Autodesk Fusion 360 part; units mm, degrees
sketch "Sketch1" plane through (0, 0, 0) normal (0, 0, 1) x (1, 0, 0)
  line L0 (-21, 20) -> (67.2, 20)
  line L1 (67.2, 20) -> (67.2, -83.2)
  line L2 (67.2, -83.2) -> (-21, -83.2)
  line L3 (-21, -83.2) -> (-21, 20)
  line L4 (-24, 23) -> (70.2, 23)
  line L5 (70.2, 23) -> (70.2, -86.2)
  line L6 (70.2, -86.2) -> (-24, -86.2)
  line L7 (-24, -86.2) -> (-24, 23)
  line L8 (-21, 20) -> (-24, 20)
  line L9 (-24, 20) -> (-24, -6.1)
  line L10 (-24, -6.1) -> (-21, -6.1)
  line L11 (-21, -6.1) -> (-21, 20)
  line L12 (-21, 20) -> (-18, 20)
  line L13 (-18, 20) -> (-18, 17)
  line L14 (-18, 17) -> (-21, 17)
  line L15 (-21, 17) -> (-21, 20)
  line L16 (67.2, 20) -> (64.2, 20)
  line L17 (64.2, 20) -> (64.2, 17)
  line L18 (64.2, 17) -> (67.2, 17)
  line L19 (67.2, 17) -> (67.2, 20)
  line L20 (-21, -83.2) -> (-18, -83.2)
  line L21 (-18, -83.2) -> (-18, -80.2)
  line L22 (-18, -80.2) -> (-21, -80.2)
  line L23 (-21, -80.2) -> (-21, -83.2)
  line L24 (67.2, -83.2) -> (64.2, -83.2)
  line L25 (64.2, -83.2) -> (64.2, -80.2)
  line L26 (64.2, -80.2) -> (67.2, -80.2)
  line L27 (67.2, -80.2) -> (67.2, -83.2)
  line L28 (-24, 20) -> (-21, 20)
  line L29 (-21, 20) -> (-21, 17)
  line L30 (-21, 17) -> (-24, 17)
  line L31 (-24, 17) -> (-24, 20)
  dimension "d1" = 88.2
  dimension "d2" = 103.2
  dimension "d3" = 94.2
  dimension "d4" = 109.2
  dimension "d5" = 3
  dimension "d6" = 3
  dimension "d7" = 3
  dimension "d8" = 26.1
  dimension "d9" = 3
  dimension "d10" = 3
  dimension "d11" = 3
  dimension "d12" = 3
  dimension "d13" = 3
  dimension "d14" = 3
  dimension "d15" = 3
  dimension "d16" = 3
extrude "Extrude1" add sketch "Sketch1" against normal blind 2 makes body 1
extrude "Extrude2" add sketch "Sketch1" along normal blind 6.4 separate body contours L0 L3 L11 L12 L13 L14 L15 L29 | L0 L1 L16 L17 L18 L19 | L2 L3 L20 L21 L22 L23 | L1 L2 L24 L25 L26 L27 makes body 2 at (65.2, 20, 2.1333) makes body 3 at (-18, -82.2, 2.1333) makes body 4 at (-20, 20, 2.1333) makes body 5 at (67.2, -81.2, 2.1333)
extrude "Extrude3" add sketch "Sketch1" along normal blind 12.5 contours L0 L1 L2 L3 L4 L5 L6 L7 L8 L10 L12 L16 L19 L20 L23 L24 L27 L28 bodies 1 2 3 4 5
extrude "Extrude4" add sketch "Sketch1" along normal blind 12.5 separate body contours L3 L7 L8 L9 L11 L15 L28 L29 L30 L31 makes body 6
fillet "Fillet1" radius 3 4 edges at (-24, -86.2, 5.25) (70.2, -86.2, 5.25) (70.2, 23, 5.25) (-24, 23, 5.25) on bodies 1
fillet "Fillet2" radius 2 1 edges at (-18, 17, 3.2) on bodies 1
fillet "Fillet3" radius 2 3 edges at (64.2, 17, 3.2) (64.2, -80.2, 3.2) (-18, -80.2, 3.2) on bodies 1
extrude "Extrude5" add sketch "Sketch1" along normal blind 2 contours L3 L7 L9 L10 L11 L30 bodies 1 6
fillet "Fillet4" radius 2 2 edges at (-22.5, 17, 2) (-22.5, -6.1, 2) on bodies 1
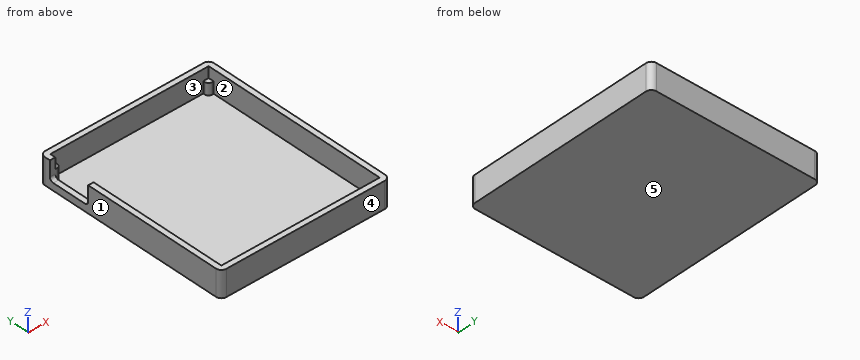
The listing builds one solid part. Answer for the finished solid, in the listing's coordinates (mm). Face numbers are marked on the shaded views. A direction names the side the tool comes from. Coordinates: 2 decimals unless noted, no trailing zeros. Write each loop counter-clockwise with the first axis right and the second up, starting at its lowest first coordinate (ties: lowest second). Pieces come first, ordered by that corner, then holes. Notation, with made-up numbers: M 43,-39.5 L 100,-39.5 A38 cw 100,-0.5 Z; hole C -23,54 d3. An arc over 180 degrees is marked long. Use a Markdown table: item, result. Add a question column.
1. Section B-B (x = 16) is taken. Give the vertices of the cut face in (y, z), plus the area to 3 significant figures.
2. For a pull along Y with two mould halves and no side action, classify the marked faces 3, 4 and 5 as +Y half, -Y half, draft (parallel to the pull), parting line (faces both ways), or undercut.
3. Section A-A (z = 8) is taken. Give the vertices of the cut face in (x, y).
4. Which of the six approach directions +Z, -Z, +X, -X, +Y, -Y give full straight-line access (tool end or side, diameter ignored) to the marked faces 1 and 2?
5. Section C-C (y = -56) is taken. Give the vertices of the cut face in (x, z), plus the area to 3 significant figures.
6. Straight lines are drawn through the part: line 1 along Y through (x, z) = (46, 6); line 2 along X through (y, z) = (-6, 1.25); line 3 along Y through (x, z) = (66, 3.5). For each, find the intervals that lie inside material, in ascending order. Write a range as [from, to].
7. Given P1, Ø3.5, axis at x = -22, y = 1, coming from the +Z side; P2, Ø0.9, axis at x = 65, y = -81.5, coming from the +Z side; P3, Ø3, axis at x = 52.5, y = -44.5, coming from the +Z side, each flat-ended and moving along its own axis, determine where each tip first touches the part or whether it passes through.
Data:
| question | item | result |
|---|---|---|
| 1 | outline | M -86.2,-2 L 23,-2 L 23,12.5 L 20,12.5 L 20,0 L -83.2,0 L -83.2,12.5 L -86.2,12.5 Z |
| 1 | area | 293 mm2 |
| 2 | face 3 | undercut |
| 2 | face 4 | -Y half |
| 2 | face 5 | draft |
| 3 | outline | M -24,-83.2 A3 ccw -21,-86.2 L 67.2,-86.2 A3 ccw 70.2,-83.2 L 70.2,20 A3 ccw 67.2,23 L -21,23 A3 ccw -24,20 L -24,17 L -21,17 L -21,20 L 67.2,20 L 67.2,-83.2 L -21,-83.2 L -21,-6.1 L -24,-6.1 Z |
| 4 | face 1 | +Z, -Z, -X, +Y, -Y |
| 4 | face 2 | +Z |
| 5 | outline | M -24,-2 L 70.2,-2 L 70.2,12.5 L 67.2,12.5 L 67.2,0 L -21,0 L -21,12.5 L -24,12.5 Z |
| 5 | area | 263 mm2 |
| 6 | line 1 | y = [-86.2, -83.2], [20, 23] |
| 6 | line 2 | x = [-24, -21], [67.2, 70.2] |
| 6 | line 3 | y = [-86.2, -80.21], [17.01, 23] |
| 7 | P1 | stops at z = 2 |
| 7 | P2 | stops at z = 6.4 |
| 7 | P3 | stops at z = 0 |
